from build123d import *

# Parameters (mm, degrees)
SKETCH1_R      = 3.4
EXTRUDE1_DEPTH = 1290
EXTRUDE2_DEPTH = 1291.174406815


with BuildPart() as part:
    # Sketch1 → Extrude1 (new body)
    with BuildSketch(Plane.XY):
        with BuildLine():
            Line((-5.1, 14.2), (-5.1, 15))
            Line((-5.1, 15), (-12.5, 15))
            ThreePointArc((-12.5, 15), (-14.267766953, 14.267766953), (-15, 12.5))
            Line((-15, 12.5), (-15, 5.1))
            Line((-15, 5.1), (-14.2, 5.1))
            Line((-14.2, 5.1), (-14.2, 4.1))
            Line((-14.2, 4.1), (-13.2, 4.1))
            Line((-13.2, 4.1), (-13.2, 8.25))
            Line((-13.2, 8.25), (-9.522792206, 8.25))
            Line((-9.522792206, 8.25), (-5.7, 4.427207794))
            Line((-5.7, 4.427207794), (-5.7, -4.427207794))
            Line((-5.7, -4.427207794), (-9.522792206, -8.25))
            Line((-9.522792206, -8.25), (-13.2, -8.25))
            Line((-13.2, -8.25), (-13.2, -4.1))
            Line((-13.2, -4.1), (-14.2, -4.1))
            Line((-14.2, -4.1), (-14.2, -5.1))
            Line((-14.2, -5.1), (-15, -5.1))
            Line((-15, -5.1), (-15, -12.5))
            ThreePointArc((-15, -12.5), (-14.267766953, -14.267766953), (-12.5, -15))
            Line((-12.5, -15), (-5.1, -15))
            Line((-5.1, -15), (-5.1, -14.2))
            Line((-5.1, -14.2), (-4.1, -14.2))
            Line((-4.1, -14.2), (-4.1, -13.2))
            Line((-4.1, -13.2), (-8.25, -13.2))
            Line((-8.25, -13.2), (-8.25, -9.522792206))
            Line((-8.25, -9.522792206), (-4.427207794, -5.7))
            Line((-4.427207794, -5.7), (4.427207794, -5.7))
            Line((4.427207794, -5.7), (8.25, -9.522792206))
            Line((8.25, -9.522792206), (8.25, -13.2))
            Line((8.25, -13.2), (4.1, -13.2))
            Line((4.1, -13.2), (4.1, -14.2))
            Line((4.1, -14.2), (5.1, -14.2))
            Line((5.1, -14.2), (5.1, -15))
            Line((5.1, -15), (12.5, -15))
            ThreePointArc((12.5, -15), (14.267766953, -14.267766953), (15, -12.5))
            Line((15, -12.5), (15, -5.1))
            Line((15, -5.1), (14.2, -5.1))
            Line((14.2, -5.1), (14.2, -4.1))
            Line((14.2, -4.1), (13.2, -4.1))
            Line((13.2, -4.1), (13.2, -8.25))
            Line((13.2, -8.25), (9.522792206, -8.25))
            Line((9.522792206, -8.25), (5.7, -4.427207794))
            Line((5.7, -4.427207794), (5.7, 4.427207794))
            Line((5.7, 4.427207794), (9.522792206, 8.25))
            Line((9.522792206, 8.25), (13.2, 8.25))
            Line((13.2, 8.25), (13.2, 4.1))
            Line((13.2, 4.1), (14.2, 4.1))
            Line((14.2, 4.1), (14.2, 5.1))
            Line((14.2, 5.1), (15, 5.1))
            Line((15, 5.1), (15, 12.5))
            ThreePointArc((15, 12.5), (14.267766953, 14.267766953), (12.5, 15))
            Line((12.5, 15), (5.1, 15))
            Line((5.1, 15), (5.1, 14.2))
            Line((5.1, 14.2), (4.1, 14.2))
            Line((4.1, 14.2), (4.1, 13.2))
            Line((4.1, 13.2), (8.25, 13.2))
            Line((8.25, 13.2), (8.25, 9.522792206))
            Line((8.25, 9.522792206), (4.427207794, 5.7))
            Line((4.427207794, 5.7), (-4.427207794, 5.7))
            Line((-4.427207794, 5.7), (-8.25, 9.522792206))
            Line((-8.25, 9.522792206), (-8.25, 13.2))
            Line((-8.25, 13.2), (-4.1, 13.2))
            Line((-4.1, 13.2), (-4.1, 14.2))
            Line((-4.1, 14.2), (-5.1, 14.2))
        make_face()
        with Locations(Location((0, 0, 0), (0, 0, 180))):
            Circle(SKETCH1_R, mode=Mode.SUBTRACT)
    extrude(amount=EXTRUDE1_DEPTH)

    # Sketch2 → Extrude2 (cut, through all)
    with BuildSketch(Plane.XY.offset(1290)):
        with BuildLine():
            Line((13.7, 12.7), (13.7, 10.55))
            ThreePointArc((13.7, 10.55), (13.407106781, 9.842893219), (12.7, 9.55))
            Line((12.7, 9.55), (10.55, 9.55))
            ThreePointArc((10.55, 9.55), (9.842893219, 9.842893219), (9.55, 10.55))
            Line((9.55, 10.55), (9.55, 12.7))
            ThreePointArc((9.55, 12.7), (9.842893219, 13.407106781), (10.55, 13.7))
            Line((10.55, 13.7), (12.7, 13.7))
            ThreePointArc((12.7, 13.7), (13.407106781, 13.407106781), (13.7, 12.7))
        make_face()
        with BuildLine():
            Line((-12.7, 13.7), (-10.55, 13.7))
            ThreePointArc((-10.55, 13.7), (-9.842893219, 13.407106781), (-9.55, 12.7))
            Line((-9.55, 12.7), (-9.55, 10.55))
            ThreePointArc((-9.55, 10.55), (-9.842893219, 9.842893219), (-10.55, 9.55))
            Line((-10.55, 9.55), (-12.7, 9.55))
            ThreePointArc((-12.7, 9.55), (-13.407106781, 9.842893219), (-13.7, 10.55))
            Line((-13.7, 10.55), (-13.7, 12.7))
            ThreePointArc((-13.7, 12.7), (-13.407106781, 13.407106781), (-12.7, 13.7))
        make_face()
        with BuildLine():
            Line((12.7, -13.7), (10.55, -13.7))
            ThreePointArc((10.55, -13.7), (9.842893219, -13.407106781), (9.55, -12.7))
            Line((9.55, -12.7), (9.55, -10.55))
            ThreePointArc((9.55, -10.55), (9.842893219, -9.842893219), (10.55, -9.55))
            Line((10.55, -9.55), (12.7, -9.55))
            ThreePointArc((12.7, -9.55), (13.407106781, -9.842893219), (13.7, -10.55))
            Line((13.7, -10.55), (13.7, -12.7))
            ThreePointArc((13.7, -12.7), (13.407106781, -13.407106781), (12.7, -13.7))
        make_face()
        with BuildLine():
            Line((-13.7, -12.7), (-13.7, -10.55))
            ThreePointArc((-13.7, -10.55), (-13.407106781, -9.842893219), (-12.7, -9.55))
            Line((-12.7, -9.55), (-10.55, -9.55))
            ThreePointArc((-10.55, -9.55), (-9.842893219, -9.842893219), (-9.55, -10.55))
            Line((-9.55, -10.55), (-9.55, -12.7))
            ThreePointArc((-9.55, -12.7), (-9.842893219, -13.407106781), (-10.55, -13.7))
            Line((-10.55, -13.7), (-12.7, -13.7))
            ThreePointArc((-12.7, -13.7), (-13.407106781, -13.407106781), (-13.7, -12.7))
        make_face()
    extrude(amount=-EXTRUDE2_DEPTH, mode=Mode.SUBTRACT)


solid = part.part
Work out the finished part from the listing and answer in its coordinate system (mm). Give positions to 0.01 mm unless a question says otherwise; leave off trailing zeros. Use a Markdown table: item, result. Add a question column.
1) Each of these flat-tipped pins is pushed along its axis until it touches: P1, Ø1.1, axis at x = -14, z = 563, coming from the +Y side; P2, Ø1.5, axis at x = -4, y = -8, coming from the -Z side; P3, Ø1.1, axis at y = 4.5, z = 759, coming from the -X side; P4, Ø1.1, axis at x = -4.5, z = 573.5, coming from the -Y side. Where does it stop, or does it pass through?
2) The part is cut by section A-A, the plane z = 243. Count the separate pieces of the cut face and the enclosed holes in it, plus the area to 3 significant figures.
3) Consider line 1 along X through (y, z) = (6.75, 1165.5); line 2 along X through (y, z) = (-11, 274.5); line 3 along Y through (x, z) = (10, 969). Determine where each line is inside the solid, lowest interval first.
Reported:
| question | item | result |
|---|---|---|
| 1 | P1 | stops at y = 14.81 |
| 1 | P2 | passes through |
| 1 | P3 | stops at x = -14.2 |
| 1 | P4 | stops at y = -14.2 |
| 2 | separate pieces | 1 |
| 2 | enclosed holes | 5 |
| 2 | area | 291 mm^2 |
| 3 | line 1 | x = -15 to -13.2, -8.02 to -5.48, 5.48 to 8.02, 13.2 to 15 |
| 3 | line 2 | x = -15 to -13.7, -9.55 to -8.25, 8.25 to 9.55, 13.7 to 15 |
| 3 | line 3 | y = -15 to -13.54, -9.71 to -8.25, 8.25 to 9.71, 13.54 to 15 |
